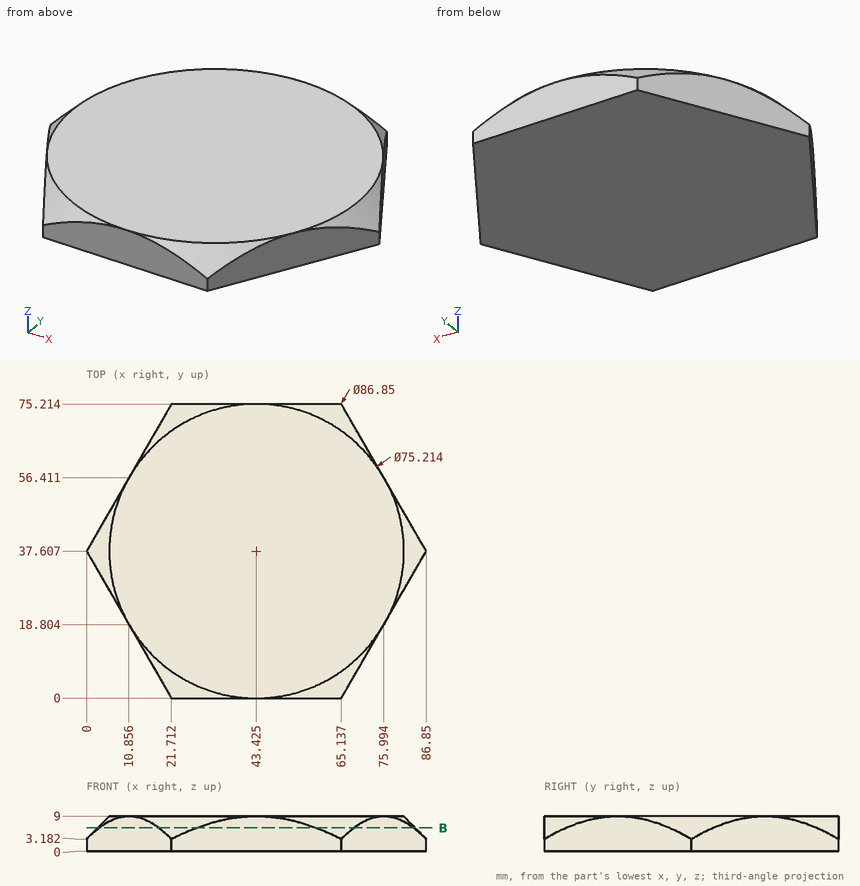
Here's the drawing with two shaded views (mm, measured from the low corner). I have some questions. Coordinates: 2 decimals unless noted, no trailing zeros. Order: outer loops, then holes, each group sorted by start corner. A loop starts at its lowest first (then second) coordinate and runs counter-clockwise, first axis right, second up.
Item 1: For P1, Ø1.5, axis at y = 57.5, z = 3.5, coming from the +X side, with a flat end and sliding along its axis, tell me the tip position at first contact or that it passes through.
Result sheet:
P1: stops at x = 75.8
Item 2: I need wall thicknesses on line 1 (X direction, y = 68.5, z = 5) (1 decimal); line 2 (X direction, y = 19.5, z = 5) (1 decimal); line 3 (Z direction, x = 17, y = 10). Which ranges of each line are inside material? Lowest first, please.
Result sheet:
line 1: x = 17.8 to 69
line 2: x = 10.5 to 76.4
line 3: z = 0 to 8.39
Item 3: If we section it at B-B on z = 6: List the corners of the cut face in (x, y) for me (1 decimal), plus the area to 3 significant figures.
Result sheet:
outline: (3.2, 32.1) - (18.5, 5.5) arc R40.6 ccw to (28.1, 0) - (58.7, 0) arc R40.6 ccw to (68.3, 5.5) - (83.7, 32.1) arc R40.6 ccw to (83.7, 43.1) - (68.3, 69.7) arc R40.6 ccw to (58.7, 75.2) - (28.1, 75.2) arc R40.6 ccw to (18.5, 69.7) - (3.2, 43.1) arc R40.6 ccw to start
area: 4,810 mm2
